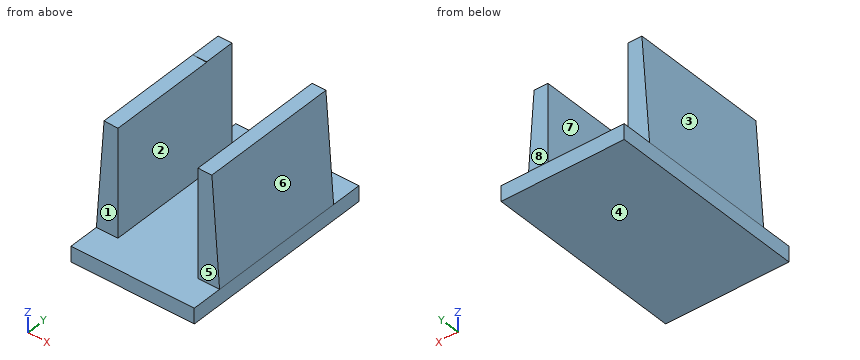
from build123d import *

# Parameters (mm, degrees)
F0_W     = 40
F0_H     = 65
F1_DEPTH = 5
F6_DEPTH = 10
F8_DEPTH = 45


with BuildPart() as f1:
    # F0 (on Top) → F1 (new body)
    with BuildSketch(Plane.XY):
        with Locations((-2.0310617983, -0.7245496807)):
            Rectangle(F0_W, F0_H)
    extrude(amount=F1_DEPTH)

    # F5 (on face) → F6 (join)
    with BuildSketch(Plane(origin=(0, 21.7754503193, 0), x_dir=(-1, 0, 0), z_dir=(0, 1, 0))):
        Polygon((15.0310617983, 40), (15.0310617983, 5), (22.0310617983, 5), (19.5310617983, 40), align=None)
        Polygon((-17.9689382017, 5), (-10.9689382017, 5), (-10.9689382017, 39.8395545781), (-15.4689382017, 40), align=None)
    extrude(amount=-F6_DEPTH)

    # F7 (on offset) → F8 (join)
    with BuildSketch(Plane.XZ.offset(23.2245496807)):
        Polygon((10.9689382017, 40), (10.9689382017, 5), (17.9689382017, 5), (15.4689382017, 40), align=None)
        Polygon((-22.0310617983, 5), (-15.0310617983, 5), (-15.0310617983, 39.8395545781), (-19.5310617983, 40), align=None)
    extrude(amount=-F8_DEPTH)


solid = f1.part
The listing builds one solid part. Answer for the finished solid, in the listing's coordinates (mm). Face numbers are marked on the shaded views. A direction names the side the tool comes from. Give positions to 0.01 mm unless a question says otherwise; leave off trailing zeros. Write each loop counter-clockwise with the first axis right and the second up, starting at its lowest first coordinate (ties: lowest second). Pieces come first, ordered by that corner, then holes. Notation, with made-up numbers: (40.25, 31.25) -> (76.25, 31.25) arc R28 cw to (76.25, 57.25) -> close; hole circle Ø11 at (-23.5, -36.75). An arc over 180 degrees is marked (long way). One line per question, with ' | ' between items. Start each with the question number.
1. Section C-C (x = -7.5) is taken. Determine the outline of the cut face in (y, z).
2. Section A-A (z = 16.5) is taken. Determine the outline of the cut face in (x, y).
3. For the marked faces 4, 5, 6, 7 and 8, determine the directions among +Z, -Z, +X, -X, +Y, -Y from which every point of the face is accessible in a straight line to the end or side of a thin tool.
4. Section B-B (y = 8.5) is taken. Determine the outline of the cut face in (x, z), plus the area to 3 significant figures.
5. Given pin 1 Ø2 at (x, z) = (-19.5, 26.5) entering from -Y; pin 2 Ø10.5 at (y, z) = (7.5, 27.5) entering from +X; pin 3 Ø2 at (x, z) = (-19, 23) entering from +Y, each flat-ended and moving along its own axis, determine where each tip first touches the part or whether it passes through.
6. Section D-D (z = 31) is taken. Determine the outline of the cut face in (x, y), plus the area to 3 significant figures.
7. For a pull along X with two mould halves and no side action, classify the marked faces 1, 2 and 3 as pulls with the +X half, pulls with the -X half, needs draft (parallel to the pull), parting line crosses it, or undercut.
8. Find the intervals of material crossed by probe 1 along Z at (x, y) = (-13.5, 3); probe 2 along X at (y, z) = (-2.5, 31); probe 3 along X at (y, z) = (-21, 8), in increasing order.
Response values:
1) outline: (-33.22, 0) -> (31.78, 0) -> (31.78, 5) -> (-33.22, 5) -> close
2) outline: (-21.21, -23.22) -> (-15.03, -23.22) -> (-15.03, 21.78) -> (-21.21, 21.78) -> close; (10.97, -23.22) -> (17.15, -23.22) -> (17.15, 21.78) -> (10.97, 21.78) -> close
3) face 4: -Z, +X, -X, +Y, -Y | face 5: +Z, +X, -X, -Y | face 6: +Z, +X, +Y, -Y | face 7: +Z, +Y, -Y | face 8: +Z, +X, -X, +Y
4) outline: (-22.03, 0) -> (17.97, 0) -> (17.97, 5) -> (15.47, 40) -> (10.97, 40) -> (10.97, 5) -> (-15.03, 5) -> (-15.03, 39.84) -> (-19.53, 40) -> (-22.03, 5) -> close | area: 602 mm2
5) pin 1: y = -23.22 | pin 2: x = 16.74 | pin 3: y = 21.78
6) outline: (-20.17, -23.22) -> (-15.03, -23.22) -> (-15.03, 21.78) -> (-20.17, 21.78) -> close; (10.97, -23.22) -> (16.11, -23.22) -> (16.11, 21.78) -> (10.97, 21.78) -> close | area: 463 mm2
7) face 1: needs draft | face 2: undercut | face 3: pulls with the -X half
8) probe 1: 0 to 5 | probe 2: -20.17 to -15.03, 10.97 to 16.11 | probe 3: -21.82 to -15.03, 10.97 to 17.75
